```python
from build123d import *

# Parameters (mm, degrees)
SKETCH1_W             = 457.2
SKETCH1_H             = 127
BOSS_EXTRUDE1_DEPTH   = 5.715
SKETCH2_W             = 19.05
SKETCH2_H             = 5.715
LED_MOUNT_HOLES_DEPTH = 6.715
SKETCH4_W             = 5.715
SKETCH4_H             = 25.4
CUT_EXTRUDE2_DEPTH    = 6.715
SKETCH5_W             = 50.8
SKETCH5_H             = 5.6642
SKETCH5_W_2           = 25.4
SKETCH5_H_2           = 5.715
CUT_EXTRUDE3_DEPTH    = 6.715
SKETCH6_W             = 0.254
SKETCH6_H             = 5.715
SKETCH6_H_2           = 5.6642
BOSS_EXTRUDE2_DEPTH   = 5.715


with BuildPart() as part:
    # Sketch1 → Boss-Extrude1 (new body)
    with BuildSketch(Plane.XY):
        Rectangle(SKETCH1_W, SKETCH1_H)
    extrude(amount=BOSS_EXTRUDE1_DEPTH)

    # Sketch2 → LED Mount Holes (cut, through all)
    with BuildSketch(Plane.XY.offset(5.715)):
        with Locations((174.625, 9.8425)):
            Rectangle(SKETCH2_W, SKETCH2_H)
        with Locations((130.175, 9.8425)):
            Rectangle(SKETCH2_W, SKETCH2_H)
    extrude(amount=-LED_MOUNT_HOLES_DEPTH, mode=Mode.SUBTRACT)

    # Sketch4 → Cut-Extrude2 (cut, through all)
    with BuildSketch(Plane(origin=(0, 0, 0), x_dir=(-1, 0, 0), z_dir=(0, 0, -1))):
        with Locations((-225.7425, 50.8)):
            Rectangle(SKETCH4_W, SKETCH4_H)
        with Locations((-225.7425, 0)):
            Rectangle(SKETCH4_W, SKETCH4_H)
        with Locations((-225.7425, -50.8)):
            Rectangle(SKETCH4_W, SKETCH4_H)
    cut_extrude2 = extrude(amount=-CUT_EXTRUDE2_DEPTH, mode=Mode.SUBTRACT)

    # Mirror1: Cut-Extrude2 across plane
    add(cut_extrude2.mirror(Plane(origin=(0, 0, 0), x_dir=(0, 0, 1), z_dir=(1, 0, 0))), mode=Mode.SUBTRACT)

    # Sketch5 → Cut-Extrude3 (cut, through all)
    with BuildSketch(Plane(origin=(0, 0, 0), x_dir=(-1, 0, 0), z_dir=(0, 0, -1))):
        with Locations((-152.4, 60.6679)):
            Rectangle(SKETCH5_W, SKETCH5_H)
        with Locations((-76.2, 60.6679)):
            Rectangle(SKETCH5_W, SKETCH5_H)
        with Locations((0, 60.6679)):
            Rectangle(SKETCH5_W, SKETCH5_H)
        with Locations((76.2, 60.6679)):
            Rectangle(SKETCH5_W, SKETCH5_H)
        with Locations((152.4, 60.6679)):
            Rectangle(SKETCH5_W, SKETCH5_H)
        with Locations((228.6, 60.6679)):
            Rectangle(SKETCH5_W, SKETCH5_H)
        with Locations((-215.9, 60.6425)):
            Rectangle(SKETCH5_W_2, SKETCH5_H_2)
    cut_extrude3 = extrude(amount=-CUT_EXTRUDE3_DEPTH, mode=Mode.SUBTRACT)

    # Sketch6 → Boss-Extrude2 (add)
    with BuildSketch(Plane(origin=(0, 0, 0), x_dir=(-1, 0, 0), z_dir=(0, 0, -1))):
        with Locations((-203.327, 60.6425)):
            Rectangle(SKETCH6_W, SKETCH6_H)
        with Locations((-177.673, 60.6425)):
            Rectangle(SKETCH6_W, SKETCH6_H)
        with Locations((-127.127, 60.6679)):
            Rectangle(SKETCH6_W, SKETCH6_H_2)
        with Locations((-101.473, 60.6679)):
            Rectangle(SKETCH6_W, SKETCH6_H_2)
        with Locations((-50.927, 60.6679)):
            Rectangle(SKETCH6_W, SKETCH6_H_2)
        with Locations((-25.273, 60.6679)):
            Rectangle(SKETCH6_W, SKETCH6_H_2)
        with Locations((25.273, 60.6679)):
            Rectangle(SKETCH6_W, SKETCH6_H_2)
        with Locations((50.927, 60.6679)):
            Rectangle(SKETCH6_W, SKETCH6_H_2)
        with Locations((101.473, 60.6679)):
            Rectangle(SKETCH6_W, SKETCH6_H_2)
        with Locations((127.127, 60.6679)):
            Rectangle(SKETCH6_W, SKETCH6_H_2)
        with Locations((177.673, 60.6679)):
            Rectangle(SKETCH6_W, SKETCH6_H_2)
        with Locations((203.327, 60.6679)):
            Rectangle(SKETCH6_W, SKETCH6_H_2)
    boss_extrude2 = extrude(amount=-BOSS_EXTRUDE2_DEPTH)

    # Mirror2: Cut-Extrude3, Boss-Extrude2 across plane
    add(cut_extrude3.mirror(Plane.ZX), mode=Mode.SUBTRACT)
    add(boss_extrude2.mirror(Plane.ZX))


solid = part.part
```
Here's how the part is built. I have some questions about the finished solid (model axes, mm). Round coordinates to 2 decimals unless told otherwise and drop trailing zeros. Order: outer loops, then holes, each group sorted by start corner. A loop starts at its lowest first (then second) coordinate and runs counter-clockwise, first axis right, second up. Notation, with made-up numbers: M 39.25,5 L 86.25,5 A17 cw 86.25,17 Z; hole C 53.5,86 d11. An arc over 180 degrees is marked long. Use CSV: the item, a comma, the result in double quotes.
1) I want a section at A-A (y = -46). List the corners of the cut face in (x, z) for me (3 decimals), then the cut area to 3 significant figures.
Taken from the geometry:
outline,"M -222.885,0 L 222.885,0 L 222.885,5.715 L -222.885,5.715 Z"
area,"2,550 mm^2"
2) I need wall thicknesses on line 1 along X through (y, z) = (12, 0.75) (3 decimals); line 2 along Y through (x, z) = (23, 4.85); line 3 along X through (y, z) = (46, 2.9) (3 decimals). Which ranges of each line are inside material? Lowest first, please. Write a range as [from, to].
Taken from the geometry:
line 1,"[-222.885, 120.65], [139.7, 165.1], [184.15, 222.885]"
line 2,"[-57.84, 57.84]"
line 3,"[-222.885, 222.885]"
3) I want a section at C-C (x = 90). List the corners of the cut face in (y, z) for me (3 decimals), then the cut area to 3 significant figures.
Taken from the geometry:
outline,"M -57.836,0 L 57.836,0 L 57.836,5.715 L -57.836,5.715 Z"
area,"661 mm^2"
4) I'm going to push flat-ended pins straight in: P1, Ø2, axis at x = 154, y = -20, coming from the -Z side; P2, Ø3, axis at x = -210, z = 3.5, coming from the -Y side; P3, Ø3, axis at y = -59.5, z = 2.5, coming from the -X side; P4, Ø3, axis at y = 61.5, z = 1.5, coming from the +X side. Where does each tip first touch, or does it pass through?
Taken from the geometry:
P1,"z = 0"
P2,"y = -57.84"
P3,"x = -203.45"
P4,"x = 203.45"
5) I want a section at B-B (z = 1.95). Count the separate pieces of the cut face and the enclosed holes in it, then the cut area to 3 significant figures.
Taken from the geometry:
separate pieces,"1"
enclosed holes,"2"
area,"53,700 mm^2"
